Input: part model. Units: mm. Frame: model coordinates. Face numbers are marked on the shaded views. A direction names the side the tool comes from. Give positions to 0.01 mm unless a question says otherwise; leave off trailing zeros. Loops run counter-clockwise (first coordinate to the right, second up) from the corner with the lowest first, then second, coordinate; pieces in that order, holes last. Notation, with made-up numbers: (5.25, 84.25) -> (45.25, 84.25) arc R33 cw to (45.25, 115.25) -> close; hole circle Ø9 at (77, -30). An arc over 180 degrees is marked (long way). Answer in a Markdown table with one row per item. Add a question column.
```python
from build123d import *

# Parameters (mm, degrees)
SKETCH1_R           = 1.4
BOSS_EXTRUDE1_DEPTH = 40
SKETCH2_R           = 3.5
BOSS_EXTRUDE2_DEPTH = 2
FILLET2_R           = 1


with BuildPart() as part:
    # Sketch1 → Boss-Extrude1 (new body)
    with BuildSketch(Plane(origin=(0, 0, 0), x_dir=(1, 0, 0), z_dir=(0, 1, 0))):
        with Locations(Location((0, 0, 0), (0, 0, 270))):
            Circle(SKETCH1_R)
    extrude(amount=BOSS_EXTRUDE1_DEPTH)

    # Sketch2 → Boss-Extrude2 (add)
    with BuildSketch(Plane.XZ):
        with Locations(Location((0, 0, 0), (0, 0, 270))):
            Circle(SKETCH2_R)
    extrude(amount=BOSS_EXTRUDE2_DEPTH)

    # Fillet2
    fillet2_edges = [part.edges().sort_by_distance(p)[0] for p in [
        (0, 40, -1.4),
    ]]
    fillet(fillet2_edges, radius=FILLET2_R)


solid = part.part
```
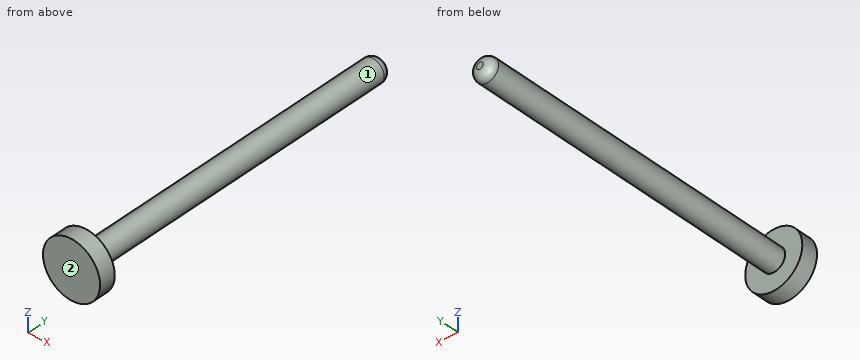
1) Reachability of the marked faces 1 and 2 from +Z, -Z, +X, -X, +Y, -Y: full face, straight path, thin tool, end or side. Return the list, or none.
2) Section A-A on y = 17. Output: boundary loops of the cut face in (x, z), and give its area (3 significant figures).
3) Section B-B on x = -3. Output: boundary loops of the cut face in (y, z).
4) Material intervals for line 1 along Y through (x, z) = (-1, 2); line 2 along X through (y, z) = (38, 0); line 3 along Z through (x, y) = (0.25, 0.5), sorted ascending.
5) Pin query (flat end, axial travel): pin 1 (4 mm diameter, centred on x = 1, y = 33, fed in from -Z); pin 2 (1.5 mm diameter, centred on y = 18, z = -1.5, fed in from -X); pin 3 (4 mm diameter, centred on x = -0.5, y = 25.5, fed in from +Z). Return the tip coordinate at first contact, or that it passes through.
Working result:
| question | item | result |
|---|---|---|
| 1 | face 1 | +Y |
| 1 | face 2 | +Z, -Z, +X, -X, -Y |
| 2 | outline | circle Ø2.8 at (0, 0) |
| 2 | area | 6.16 mm2 |
| 3 | outline | (-2, -1.8) -> (0, -1.8) -> (0, 1.8) -> (-2, 1.8) -> close |
| 4 | line 1 | y = -2 to 0 |
| 4 | line 2 | x = -1.4 to 1.4 |
| 4 | line 3 | z = -1.38 to 1.38 |
| 5 | pin 1 | stops at z = -1.4 |
| 5 | pin 2 | stops at x = -1.18 |
| 5 | pin 3 | stops at z = 1.4 |
